```python
from build123d import *

# Parameters (mm, degrees)
SKETCH1_W                = 50
SKETCH1_H                = 50
BOSS_EXTRUDE1_DEPTH      = 50
CUT_EXTRUDE1_DEPTH       = 87.602540378
CUT_EXTRUDE2_DEPTH       = 87.602540378
CHAMFER1_SIZE            = 1.5
BOSS_EXTRUDE2_DEPTH      = 7
BOSS_EXTRUDE2_DEPTH_BACK = 10
SKETCH4_W                = 1
SKETCH4_H                = 7
SKETCH5_W                = 1.8
SKETCH5_H                = 1.8
CUT_EXTRUDE3_DEPTH       = 7


with BuildPart() as part:
    # Sketch1 → Boss-Extrude1 (new body)
    with BuildSketch(Plane.XY):
        with Locations((25, 25)):
            Rectangle(SKETCH1_W, SKETCH1_H)
    extrude(amount=BOSS_EXTRUDE1_DEPTH)

    # Sketch2 → Cut-Extrude1 (cut, through all)
    with BuildSketch(Plane.ZY):
        Polygon((36, 29.556349186), (29.556349186, 36), (20.443650814, 36), (14, 29.556349186), (14, 20.443650814), (20.443650814, 14), (29.556349186, 14), (36, 20.443650814), align=None)
        Polygon((61, 29.556349186), (54.556349186, 36), (45.443650814, 36), (39, 29.556349186), (39, 20.443650814), (45.443650814, 14), (54.556349186, 14), (61, 20.443650814), align=None)
    extrude(amount=-CUT_EXTRUDE1_DEPTH, mode=Mode.SUBTRACT)

    # Sketch3 → Cut-Extrude2 (cut, through all)
    with BuildSketch(Plane.XZ):
        Polygon((29.556349186, 39), (36, 45.443650814), (36, 54.556349186), (29.556349186, 61), (20.443650814, 61), (14, 54.556349186), (14, 45.443650814), (20.443650814, 39), align=None)
    extrude(amount=-CUT_EXTRUDE2_DEPTH, mode=Mode.SUBTRACT)

    # Chamfer1
    chamfer1_edges = [part.edges().sort_by_distance(p)[0] for p in [
        (50, 7, 50),
        (0, 7, 50),
        (50, 43, 50),
        (7, 36, 50),
        (43, 14, 50),
        (43, 50, 50),
        (50, 14, 47.721825407),
        (50, 36, 47.721825407),
        (0, 14, 47.721825407),
        (0, 36, 47.721825407),
        (0, 32.778174593, 42.221825407),
        (0, 17.221825407, 42.221825407),
        (50, 17.221825407, 42.221825407),
        (50, 32.778174593, 42.221825407),
        (43, 36, 50),
        (36, 36, 47.721825407),
        (14, 36, 47.721825407),
        (7, 14, 50),
        (7, 50, 50),
        (43, 0, 50),
        (36, 0, 47.721825407),
        (14, 0, 47.721825407),
        (17.221825407, 0, 42.221825407),
        (32.778174593, 0, 42.221825407),
        (14, 7, 50),
        (14, 14, 47.721825407),
        (14, 43, 50),
        (14, 50, 47.721825407),
        (36, 14, 47.721825407),
        (36, 7, 50),
        (36, 50, 47.721825407),
        (36, 43, 50),
        (17.221825407, 50, 42.221825407),
        (32.778174593, 50, 42.221825407),
        (0, 43, 50),
        (25, 50, 0),
        (50, 25, 0),
        (25, 0, 0),
        (0, 25, 0),
        (7, 0, 50),
        (0, 50, 25),
        (50, 50, 25),
        (50, 0, 25),
        (0, 0, 25),
    ]]
    chamfer(chamfer1_edges, length=CHAMFER1_SIZE)

    # Sketch4 → Boss-Extrude2 (add, two sides: drawn at the far end of the back side and taken through both)
    with BuildSketch(Plane.XY.offset(50).offset(-BOSS_EXTRUDE2_DEPTH_BACK)):
        with Locations((49.5, 7)):
            Rectangle(SKETCH4_W, SKETCH4_H)
    extrude(amount=BOSS_EXTRUDE2_DEPTH + BOSS_EXTRUDE2_DEPTH_BACK)

    # Sketch5 → Cut-Extrude3 (cut)
    with BuildSketch(Plane(origin=(50, 0, 0), x_dir=(0, 0, -1), z_dir=(1, 0, 0))):
        with Locations((-53.6, 7)):
            Rectangle(SKETCH5_W, SKETCH5_H)
    extrude(amount=-CUT_EXTRUDE3_DEPTH, mode=Mode.SUBTRACT)


solid = part.part
```
Check sheet for the modelled part. Datum: model origin and axes. Units: mm. A direction names the side the tool comes from. Give positions to 0.01 mm unless a question says otherwise; leave off trailing zeros. Order: outer loops, then holes, each group sorted by start corner. A loop starts at its lowest first (then second) coordinate and runs counter-clockwise, first axis right, second up. Notation, with made-up numbers: (35, 7.25) -> (68, 7.25) arc R23 ccw to (68, 38.25) -> close; hole circle Ø11 at (17.25, 20). An arc over 180 degrees is marked (long way). Return JSON: item names as keys, results as strings.
1. Cross-section at B-B, the plane x = 22.5. Record the cut outline in (y, z), plus the area to 3 significant figures.
From the geometry:
{"outline": "(0, 1.5) -> (1.5, 0) -> (48.5, 0) -> (50, 1.5) -> (50, 39) -> (0, 39) -> close; hole (14, 20.44) -> (20.44, 14) -> (29.56, 14) -> (36, 20.44) -> (36, 29.56) -> (29.56, 36) -> (20.44, 36) -> (14, 29.56) -> close", "area": "1,550 mm^2"}
2. Material ranges on probe 1 along Z at (x, y) = (5, 29); probe 2 along Y at (x, z) = (16.5, 24); probe 3 along Y at (x, z) = (19, 35), recorded low to high. Write a range as [from, to].
From the geometry:
{"probe 1": "[0, 14], [36, 39]", "probe 2": "[0, 14], [36, 50]", "probe 3": "[0, 19.44], [30.56, 50]"}
3. Set-up check for faces 5 (the flat face through (1, 13, 49)), 6 (the flat face through (37, 49, 49)), 7 (the flat face through (49.24, 33.57, 41.97)): record each of +Z, -Z, +X, -X, +Y, -Y from which the full face is reachable in a straight line by a thin tool's end or side.
From the geometry:
{"face 5": "+Z, -X", "face 6": "+Z, +Y", "face 7": "+Z, +X"}
4. Cross-section at A-A, the plane z = 21.5. Record the cut outline in (x, y).
From the geometry:
{"outline": "(0, 1.5) -> (1.5, 0) -> (48.5, 0) -> (50, 1.5) -> (50, 14) -> (0, 14) -> close; (0, 36) -> (50, 36) -> (50, 48.5) -> (48.5, 50) -> (1.5, 50) -> (0, 48.5) -> close"}
5. Cross-section at C-C, the plane z = 47. Count the separate pieces of the cut face and the enclosed holes in it, plus the area to 3 significant figures.
From the geometry:
{"separate pieces": "4", "enclosed holes": "0", "area": "766 mm^2"}
6. Go/stop test with flat-tipped pins: P1, Ø5, axis at x = 39.5, y = 11, coming from the +Z side; P2, Ø7.5, axis at x = 24.5, y = 25.5, coming from the +Z side; P3, Ø10, axis at y = 20.5, z = 30, coming from the +X side; P4, Ø0.5, axis at x = 49.5, z = 51, coming from the +Y side. Record where each tip stops, or that it passes through.
From the geometry:
{"P1": "z = 50", "P2": "z = 39", "P3": "x = 50", "P4": "y = 10.5"}
7. Cross-section at D-D, the plane y = 34. Record the cut outline in (x, z), plus the area to 3 significant figures.
From the geometry:
{"outline": "(0, 1.5) -> (1.5, 0) -> (48.5, 0) -> (50, 1.5) -> (50, 18.44) -> (0, 18.44) -> close; (0, 31.56) -> (50, 31.56) -> (50, 41.32) -> (48.5, 43.44) -> (34, 43.44) -> (29.56, 39) -> (20.44, 39) -> (16, 43.44) -> (1.5, 43.44) -> (0, 41.32) -> close", "area": "1,450 mm^2"}
8. Mould release check, pull along X, two halves, no side actions. Record for faces 1 (the flat face through (36.7, 0.8, 46.6)), 2 (the flat face through (7, 7, 50)), 3 (the flat face through (14, 43, 47)), 4 (the flat face through (1, 1, 1)): +X half, -X half, draft (parallel to the pull), parting line (faces both ways), or undercut.
From the geometry:
{"face 1": "undercut", "face 2": "draft", "face 3": "undercut", "face 4": "-X half"}
